Check sheet for the drawn part. Datum: minimum x, y, z corner. Units: mm. Coordinates: 2 decimals unless noted, no trailing zeros. Answer as CSV lines item,"result". Start each with the question number.
Q1. Sectioned sample at A-A, the plane y = 16. Count the separate pieces of the cut face and the enclosed holes in it, then the cut area to 3 significant figures.
Q2. Depth check by flat-ended pin: pin 1 Ø20 at (x, z) = (31, 31) entering from -Y; pin 2 Ø3 at (y, z) = (25, 22.5) entering from +X; pin 3 Ø5 at (x, y) = (36, 20) entering from +Z; pin 4 Ø8 at (y, z) = (26.5, 43.5) entering from -X. Enter the tip coordinate at first touch or a pass-through.
Q3. Thickness scan on line 1 along X through (y, z) = (9.75, 31); line 2 along Z through (x, y) = (19, 20.5) (1 decimal); line 3 along X through (y, z) = (20.5, 26) (1 decimal). Record the ranges inside material, lowest first. Write a range as from..to.
Q4. Mould release check, pull along X, two halves, no side actions. Record for the marked faces 1, 2, 3 and 4: pulls with the +X half, pulls with the -X half, needs draft (parallel to the pull), parting line crosses it, or undercut.
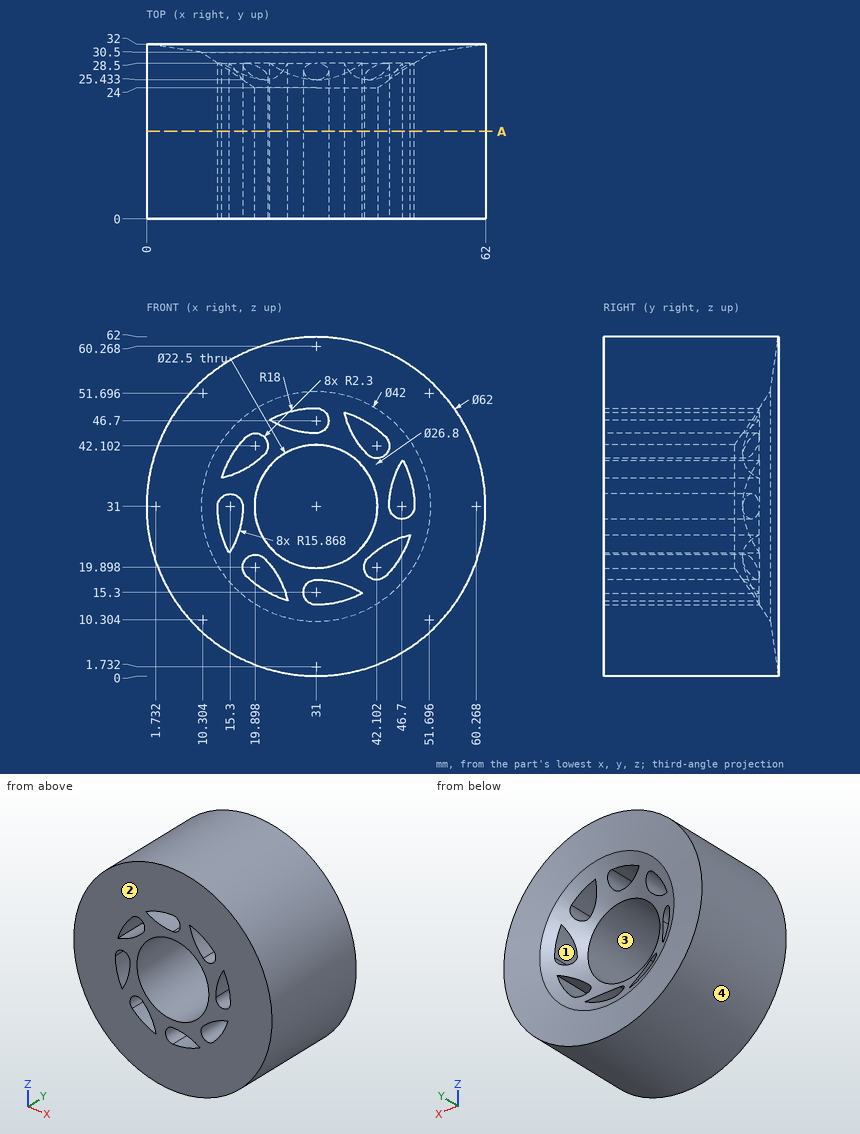
Output:
1,separate pieces,"1"
1,enclosed holes,"9"
1,area,"2,340 mm^2"
2,pin 1,"passes through"
2,pin 2,"stops at x = 61.2"
2,pin 3,"stops at z = 61.9"
2,pin 4,"stops at x = 1.19"
3,line 1,"x = 0..13, 17.6..19.75, 42.25..44.4, 49..62"
3,line 2,"z = 2.4..17.6, 22..38.4, 44.2..59.6"
3,line 3,"x = 0.4..13.7, 16.8..20.9, 41.1..61.6"
4,face 1,"undercut"
4,face 2,"needs draft"
4,face 3,"undercut"
4,face 4,"parting line crosses it"
